Source: CAD feature listing. Evaluate the final solid. Frame: model axes, mm. Face numbers are marked on the shaded views. Give positions to 0.01 mm unless a question says otherwise; leave off trailing zeros. Loops run counter-clockwise (first coordinate to the right, second up) from the corner with the lowest first, then second, coordinate; pieces in that order, holes last. Notation, with made-up numbers: M 71,39.25 L 81,39.25 A37 ccw 81,78.25 Z; hole C -24,69 d11. An arc over 180 degrees is marked long. Answer in a Markdown table with one row per item.
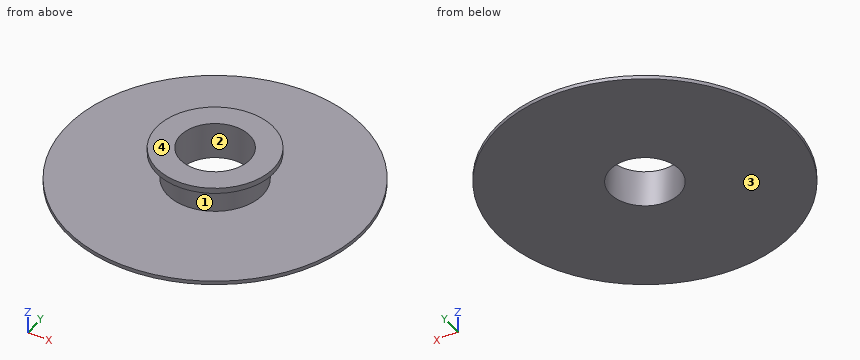
```python
from build123d import *

# Parameters (mm, degrees)
SKETCH1_R           = 81
SKETCH1_R_2         = 19
BOSS_EXTRUDE1_DEPTH = 2
SKETCH2_R           = 26
SKETCH2_R_2         = 19
BOSS_EXTRUDE2_DEPTH = 18
BOSS_EXTRUDE3_START = -3
SKETCH3_R           = 32
SKETCH3_R_2         = 26
BOSS_EXTRUDE3_DEPTH = 3


with BuildPart() as part:
    # Sketch1 → Boss-Extrude1 (new body)
    with BuildSketch(Plane.XY):
        Circle(SKETCH1_R)
        Circle(SKETCH1_R_2, mode=Mode.SUBTRACT)
    extrude(amount=BOSS_EXTRUDE1_DEPTH)

    # Sketch2 → Boss-Extrude2 (add)
    with BuildSketch(Plane.XY.offset(2)):
        Circle(SKETCH2_R)
        Circle(SKETCH2_R_2, mode=Mode.SUBTRACT)
    extrude(amount=BOSS_EXTRUDE2_DEPTH)

    # Sketch3 → Boss-Extrude3 (add)
    with BuildSketch(Plane.XY.offset(20).offset(BOSS_EXTRUDE3_START)):
        Circle(SKETCH3_R)
        Circle(SKETCH3_R_2, mode=Mode.SUBTRACT)
    extrude(amount=BOSS_EXTRUDE3_DEPTH)


solid = part.part
```
1) Section A-A, the plane y = 0. Return loops of the section in (x, z).
Reply:
| item | result |
|---|---|
| outline | M -81,0 L -19,0 L -19,20 L -32,20 L -32,17 L -26,17 L -26,2 L -81,2 Z; M 19,0 L 81,0 L 81,2 L 26,2 L 26,17 L 32,17 L 32,20 L 19,20 Z |
2) Section C-C, the plane z = 12. Return loops of the section in (x, y), then the cut area to 3 significant figures.
Reply:
| item | result |
|---|---|
| outline | C 0,0 d52; hole C 0,0 d38 |
| area | 990 mm² |
3) Section D-D, the plane y = -28. Return loops of the section in (x, z).
Reply:
| item | result |
|---|---|
| outline | M -76.01,0 L 76.01,0 L 76.01,2 L -76.01,2 Z; M -15.49,17 L 15.49,17 L 15.49,20 L -15.49,20 Z |
4) Pin query (flat end, axial travel): pin 1 Ø5 at (y, z) = (-43, 4) entering from -X; pin 2 Ø1.5 at (x, y) = (-55, -58.5) entering from -Z; pin 3 Ø19 at (x, y) = (8, 2.5) entering from -Z; pin 4 Ø2 at (y, z) = (17.5, 13.5) entering from +X. Return the tip coordinate at first contact, or that it passes through.
Reply:
| item | result |
|---|---|
| pin 1 | stops at x = -69.56 |
| pin 2 | stops at z = 0 |
| pin 3 | passes through |
| pin 4 | stops at x = 20.09 |
5) Material intervals for L1, parallel to Y at x = 0, z = 6.5; L2, parallel to Z at x = 46.5, y = 6.5; L3, parallel to Z at x = 15, y = 28, sorted ascending.
Reply:
| item | result |
|---|---|
| L1 | y = -26 to -19, 19 to 26 |
| L2 | z = 0 to 2 |
| L3 | z = 0 to 2, 17 to 20 |
6) Pull-direction query (Z, two-part tool) for the marked faces 1, 2, 3 and 4; classes: released by +Z, released by -Z, zero draft, split by the parting line, or undercut.
Reply:
| item | result |
|---|---|
| face 1 | undercut |
| face 2 | zero draft |
| face 3 | released by -Z |
| face 4 | released by +Z |
